Verification items for this drawing (mm, ordinates from the low corner). A direction names the side the tool comes from. Give positions to 0.01 mm unless a question says otherwise; leave off trailing zeros. Loops run counter-clockwise (first coordinate to the right, second up) from the corner with the lowest first, then second, coordinate; pieces in that order, holes last. Notation, with made-up numbers: M 54.25,20.25 L 92.25,20.25 A15 ccw 92.25,38.25 Z; hole C 74,27 d9. An arc over 180 degrees is marked long. Answer in a Markdown table with one row per item.
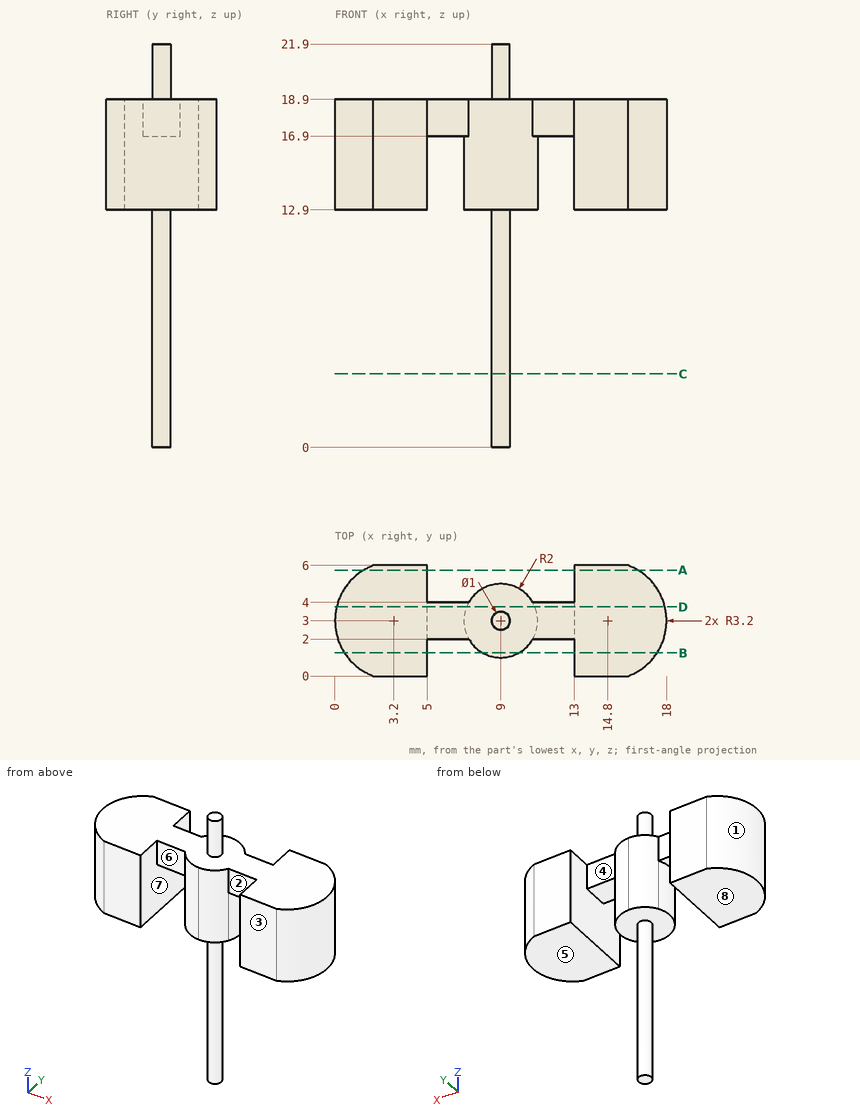
Item 1: Tool access check on the marked faces 4, 5, 6, 7 and 8. Record the directions out of +Z, -Z, +X, -X, +Y, -Y that give a thin tool (end or side, any length) a straight path to the whole face; none if there is none.
Reported:
| item | result |
|---|---|
| face 4 | +Z, -Z, +Y |
| face 5 | -Z, +X, +Y, -Y |
| face 6 | +Z, -Z, -Y |
| face 7 | -Z |
| face 8 | -Z, -X, +Y, -Y |
Item 2: Release check for a two-part mould opening along X. For the marked faces 1, 2 and 3 record: released by +X, released by -X, zero draft, split by the parting line, or undercut.
Reported:
| item | result |
|---|---|
| face 1 | released by -X |
| face 2 | undercut |
| face 3 | zero draft |
Item 3: Scan lines: L1, parallel to X at y = 4.5, z = 17.5; L2, parallel to Z at x = 14, y = 0.75; L3, parallel to X at y = 1.75, z = 13. Record each from-to range of solid material in increasing order. Write a range as [from, to].
Reported:
| item | result |
|---|---|
| L1 | x = [0.37, 5], [7.68, 10.32], [13, 17.63] |
| L2 | z = [12.9, 18.9] |
| L3 | x = [0.25, 5], [7.44, 10.56], [13, 17.75] |
Item 4: Sectioned sample at A-A (y = 5.75). Record the cut outline in (x, z).
Reported:
| item | result |
|---|---|
| outline | M 1.56,12.9 L 5,12.9 L 5,18.9 L 1.56,18.9 Z; M 13,12.9 L 16.44,12.9 L 16.44,18.9 L 13,18.9 Z |
Item 5: Go/stop test with flat-tipped pins: pin 1 (2 mm diameter, centred on y = 1, z = 18, fed in from -X); pin 2 (1.5 mm diameter, centred on x = 16.5, y = 3, fed in from -Z); pin 3 (2 mm diameter, centred on x = 11.5, z = 18, fed in from +Y). Record where each tip stops, or that it passes through.
Reported:
| item | result |
|---|---|
| pin 1 | stops at x = 0.16 |
| pin 2 | stops at z = 12.9 |
| pin 3 | stops at y = 4.32 |
Item 6: Sectioned sample at B-B (y = 1.25). Record the cut outline in (x, z).
Reported:
| item | result |
|---|---|
| outline | M 0.52,12.9 L 5,12.9 L 5,18.9 L 0.52,18.9 Z; M 8.03,12.9 L 9.97,12.9 L 9.97,18.9 L 8.03,18.9 Z; M 13,12.9 L 17.48,12.9 L 17.48,18.9 L 13,18.9 Z |
Item 7: Sectioned sample at D-D (y = 3.75). Record the cut outline in (x, z), and give its area (3 significant figures).
Reported:
| item | result |
|---|---|
| outline | M 0.09,12.9 L 5,12.9 L 5,16.9 L 7.15,16.9 L 7.15,12.9 L 10.85,12.9 L 10.85,16.9 L 13,16.9 L 13,12.9 L 17.91,12.9 L 17.91,18.9 L 0.09,18.9 Z |
| area | 89.8 mm^2 |
Item 8: Sectioned sample at C-C (z = 4). Record the cut outline in (x, y), and give its area (3 significant figures).
Reported:
| item | result |
|---|---|
| outline | C 9,3 d1 |
| area | 0.785 mm^2 |
